Input: part model. Units: mm. Frame: model coordinates. Face numbers are marked on the shaded views. Coordinates: 2 decimals unless noted, no trailing zeros. Write each loop counter-clockwise with the first axis right and the second up, starting at its lowest first coordinate (ties: lowest second). Pieces come first, ordered by that corner, then holes.
from build123d import *

# Parameters (mm, degrees)
CROQUIS1_W              = 240
CROQUIS1_H              = 90
CROQUIS1_R              = 17.5
CROQUIS1_R_2            = 16.5
SALIENTE_EXTRUIR1_DEPTH = 10
CORTAR_EXTRUIR1_DEPTH   = 5


with BuildPart() as part:
    # Croquis1 → Saliente-Extruir1 (new body)
    with BuildSketch(Plane.XY):
        with Locations((120, 45)):
            Rectangle(CROQUIS1_W, CROQUIS1_H)
        with Locations((120, 45)):
            Circle(CROQUIS1_R, mode=Mode.SUBTRACT)
        with Locations((40, 45)):
            Circle(CROQUIS1_R_2, mode=Mode.SUBTRACT)
        with Locations(Location((200, 45, 0), (0, 0, 180))):
            Circle(CROQUIS1_R_2, mode=Mode.SUBTRACT)
    extrude(amount=SALIENTE_EXTRUIR1_DEPTH)

    # Croquis2 → Cortar-Extruir1 (cut)
    with BuildSketch(Plane(origin=(0, 0, 0), x_dir=(-1, 0, 0), z_dir=(0, 0, -1))):
        with BuildLine():
            Line((-120, 62.5), (-120, 67.5))
            Line((-120, 67.5), (-165, 67.5))
            Line((-165, 67.5), (-165, 22.5))
            Line((-165, 22.5), (-120, 22.5))
            Line((-120, 22.5), (-120, 27.5))
            ThreePointArc((-120, 27.5), (-137.5, 45), (-120, 62.5))
        make_face()
    extrude(amount=-CORTAR_EXTRUIR1_DEPTH, mode=Mode.SUBTRACT)


solid = part.part
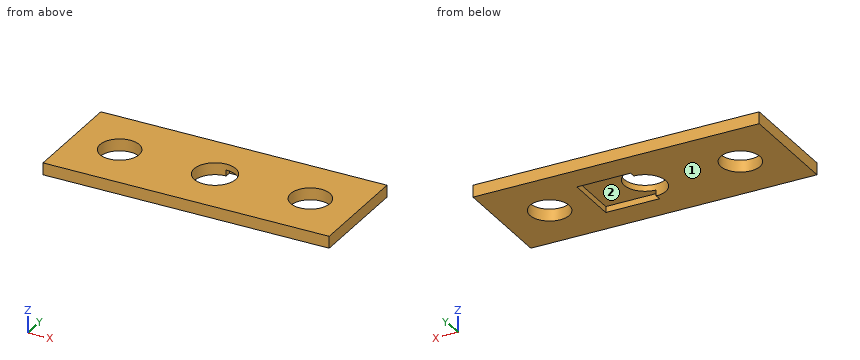
Item 1: Section query B-B, the plane x = 200. Return loops of the section in (y, z).
Item 2: Section query A-A, the plane y = 45. Return loops of the section in (x, z), then the cut area to 3 significant figures.
Item 3: Section query D-D, the plane y = 65. Return loops of the section in (x, z).
Item 4: Pin query (flat end, axial travel): pin 1 Ø6 at (x, y) = (62, 16) entering from -Z. Return the tip coordinate at first contact, or that it passes through.
Item 5: Material intervals for line 1 (Y direction, x = 120, z = 7.75); line 2 (X direction, y = 41.5, z = 6.5); line 3 (X direction, y = 34, z = 5.5), sorted ascending.
Item 6: Section query C-C, the plane z = 1.75. Return loops of the section in (x, y), then the cut area to 3 significant figures.
Item 7: Pull-direction query (X, two-part tool) for the marked faces 1 and 2; classes: released by +X, released by -X, zero draft, split by the parting line, or undercut.
The answers:
1. outline: (0, 0) - (28.5, 0) - (28.5, 10) - (0, 10) - close; (61.5, 0) - (90, 0) - (90, 10) - (61.5, 10) - close
2. outline: (0, 0) - (23.5, 0) - (23.5, 10) - (0, 10) - close; (56.5, 0) - (102.5, 0) - (102.5, 10) - (56.5, 10) - close; (137.5, 5) - (165, 5) - (165, 0) - (183.5, 0) - (183.5, 10) - (137.5, 10) - close; (216.5, 0) - (240, 0) - (240, 10) - (216.5, 10) - close
2. area: 1,250 mm2
3. outline: (0, 0) - (120, 0) - (120, 5) - (165, 5) - (165, 0) - (240, 0) - (240, 10) - (0, 10) - close
4. pin 1: stops at z = 0
5. line 1: y = 0 to 27.5, 62.5 to 90
5. line 2: x = 0 to 23.88, 56.12 to 102.85, 137.15 to 183.88, 216.12 to 240
5. line 3: x = 0 to 27.7, 52.3 to 106.39, 133.61 to 187.7, 212.3 to 240
6. outline: (0, 0) - (240, 0) - (240, 90) - (0, 90) - close; hole circle Ø33 at (40, 45); hole (120, 22.5) - (165, 22.5) - (165, 67.5) - (120, 67.5) - (120, 62.5) arc R17.5 ccw to (120, 27.5) - close; hole circle Ø33 at (200, 45)
6. area: 17,400 mm2
7. face 1: zero draft
7. face 2: undercut
